Part model, mm, in its own coordinate system. Face numbers are marked on the shaded views. A direction names the side the tool comes from. Give positions to 0.01 mm unless a question says otherwise; leave off trailing zeros. Write each loop counter-clockwise with the first axis right and the second up, starting at its lowest first coordinate (ties: lowest second). Pieces come first, ordered by that corner, then holes. Notation, with made-up numbers: M 31.25,-18 L 83.25,-18 A29 ccw 83.25,18 Z; hole C -0.75,68.25 d9. An arc over 180 degrees is marked long. Use a Markdown table: item, result.
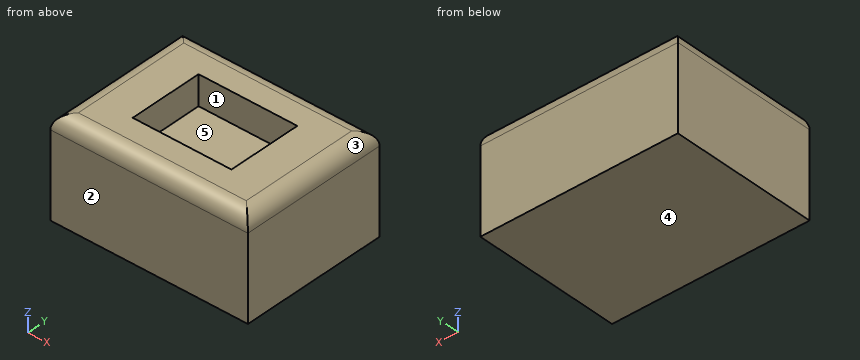
```python
from build123d import *

# Parameters (mm, degrees)
SKETCH_1_W      = 40
SKETCH_1_H      = 30
M0_BOSS_DEPTH   = 20
SKETCH_2_W      = 20
SKETCH_2_H      = 15
M0_POCKET_DEPTH = 6
M0_TOPR3_R      = 3


with BuildPart() as part:
    # ｽｹｯﾁ1 → M0_Boss (new body)
    with BuildSketch(Plane.XY):
        Rectangle(SKETCH_1_W, SKETCH_1_H)
    extrude(amount=M0_BOSS_DEPTH)

    # ｽｹｯﾁ2 → M0_Pocket (cut)
    with BuildSketch(Plane.XY.offset(20)):
        Rectangle(SKETCH_2_W, SKETCH_2_H)
    extrude(amount=-M0_POCKET_DEPTH, mode=Mode.SUBTRACT)

    # M0_TopR3
    m0_topr3_edges = [part.edges().sort_by_distance(p)[0] for p in [
        (20, 0, 20),
        (0, 15, 20),
        (-20, 0, 20),
        (0, -15, 20),
    ]]
    fillet(m0_topr3_edges, radius=M0_TOPR3_R)


solid = part.part
```
1. Cut at B-B, the plane x = -3.5. Give the cut face in (y, z), then the cut area to 3 significant figures.
Findings below:
| item | result |
|---|---|
| outline | M -15,0 L 15,0 L 15,17 A3 ccw 12,20 L 7.5,20 L 7.5,14 L -7.5,14 L -7.5,20 L -12,20 A3 ccw -15,17 Z |
| area | 506 mm2 |
2. Cut at A-A, the plane y = -0.75. Give the cut face in (x, z), then the cut area to 3 significant figures.
Findings below:
| item | result |
|---|---|
| outline | M -20,0 L 20,0 L 20,17 A3 ccw 17,20 L 10,20 L 10,14 L -10,14 L -10,20 L -17,20 A3 ccw -20,17 Z |
| area | 676 mm2 |
3. Two-plate mould, pull along X, no slides. Class the marked faces 1, 2 and 3: released by +X, released by -X, zero draft, split by the parting line, or undercut.
Findings below:
| item | result |
|---|---|
| face 1 | undercut |
| face 2 | zero draft |
| face 3 | released by +X |
4. Drill centre lines: L1, parallel to Y at x = -8, z = 16.5; L2, parallel to Z at x = 2, y = 2; L3, parallel to X at y = -1, z = 18.75. Where is each one in solid material? Low to high.
Findings below:
| item | result |
|---|---|
| L1 | -15 to -7.5, 7.5 to 15 |
| L2 | 0 to 14 |
| L3 | -19.44 to -10, 10 to 19.44 |
5. Tool access for the marked faces 4 and 5: list every direction of +Z, -Z, +X, -X, +Y, -Y with a clear straight run to the whole face (end or side of a thin tool).
Findings below:
| item | result |
|---|---|
| face 4 | -Z, +X, -X, +Y, -Y |
| face 5 | +Z |
6. Cut at C-C, the plane z = 18.25. Give the cut face in (x, y).
Findings below:
| item | result |
|---|---|
| outline | M -19.73,-14.73 L 19.73,-14.73 L 19.73,14.73 L -19.73,14.73 Z; hole M -10,-7.5 L 10,-7.5 L 10,7.5 L -10,7.5 Z |
7. Drop flat-ended pins along their axis: P1, Ø8, axis at x = -2, y = -7, coming from the +Z side; P2, Ø10, axis at x = 4.5, y = -0.5, coming from the +Z side. Give the stop position or say it passes through.
Findings below:
| item | result |
|---|---|
| P1 | z = 20 |
| P2 | z = 14 |
